Can you work these out from the model? Positions are in its coordinate system, mm. Give positions to 0.01 mm unless a question says otherwise; leave off trailing zeros. Loops run counter-clockwise (first coordinate to the right, second up) from the corner with the lowest first, then second, coordinate; pieces in that order, holes last. Notation, with made-up numbers: (15.5, 84) - (57.5, 84) arc R25 ccw to (57.5, 108) - close; hole circle Ø9 at (59.25, -10.75). An arc over 180 degrees is marked (long way). Use a Markdown table: item, result. Add a question column.
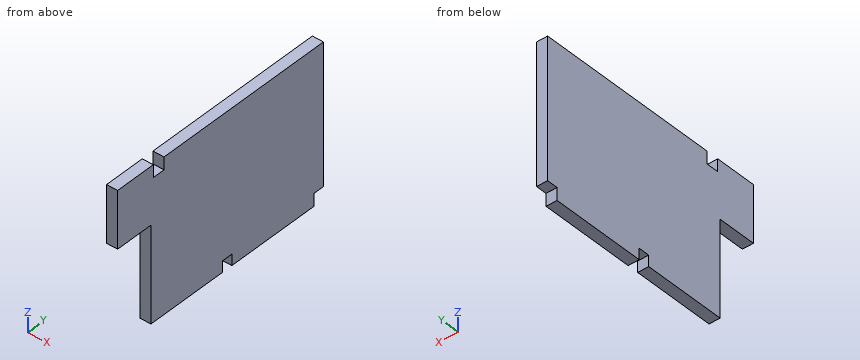
```python
from build123d import *

# Parameters (mm, degrees)
F1_DEPTH = 10.16


with BuildPart() as f1:
    # F0 (on Right) → F1 (new body)
    with BuildSketch(Plane.YZ):
        Polygon((-33.151075, -29.448999), (-43.265525, -29.448999), (-203.323364, -29.448999), (-203.323364, -40.867418), (-214.765817, -40.867418), (-214.765817, -29.448999), (-252.887964, -29.448999), (-252.887964, -81.55378), (-217.317522, -81.55378), (-217.317522, -169.236988), (-141.089514, -169.236988), (-141.089514, -159.098729), (-130.937725, -159.098729), (-130.937725, -169.236988), (-43.265525, -169.236988), (-43.265525, -157.767057), (-33.151075, -157.767057), align=None)
    extrude(amount=F1_DEPTH)


solid = f1.part
```
1. Suppose I cut it at B-B (z = -153). List the corners of the cut face in (x, y) for me.
2. Will this pin go through, and if not, where does the flat tip stop? P1, Ø3, axis at x = 5.5, z = -111, coming from the -Y side.
3. Suppose I cut it at A-A (x = 7). List the corners of the cut face in (y, z) for me.
4. Please list where these lines run through material, in increasing order: line 1 along Y through (x, z) = (4.25, -160.5); line 2 along Y through (x, z) = (9.5, -146); line 3 along Z through (x, y) = (3.5, -234). Write a range as [from, to].
Results below:
| question | item | result |
|---|---|---|
| 1 | outline | (0, -217.32) - (10.16, -217.32) - (10.16, -33.15) - (0, -33.15) - close |
| 2 | P1 | y = -217.32 |
| 3 | outline | (-252.89, -81.55) - (-217.32, -81.55) - (-217.32, -169.24) - (-141.09, -169.24) - (-141.09, -159.1) - (-130.94, -159.1) - (-130.94, -169.24) - (-43.27, -169.24) - (-43.27, -157.77) - (-33.15, -157.77) - (-33.15, -29.45) - (-203.32, -29.45) - (-203.32, -40.87) - (-214.77, -40.87) - (-214.77, -29.45) - (-252.89, -29.45) - close |
| 4 | line 1 | [-217.32, -141.09], [-130.94, -43.27] |
| 4 | line 2 | [-217.32, -33.15] |
| 4 | line 3 | [-81.55, -29.45] |
